For this review, take the finished solid that the model builds, in its own axes (mm). Round coordinates to 2 decimals unless told otherwise and drop trailing zeros. Write each loop counter-clockwise with the first axis right and the second up, starting at its lowest first coordinate (ties: lowest second). Pieces come first, ordered by that corner, then holes.
from build123d import *

# Parameters (mm, degrees)
F0_R     = 2.5
F1_DEPTH = 40


with BuildPart() as f1:
    # F0 (on Front) → F1 (new body)
    with BuildSketch(Plane.XZ):
        with BuildLine():
            Line((0, 37.70469), (0, 0))
            Line((0, 0), (60, 0))
            Line((60, 0), (60, 37.70469))
            ThreePointArc((60, 37.70469), (30, 45), (0, 37.70469))
        make_face()
        with Locations((7.5, 34)):
            Circle(F0_R, mode=Mode.SUBTRACT)
        with Locations((52.5, 34)):
            Circle(F0_R, mode=Mode.SUBTRACT)
    extrude(amount=F1_DEPTH)


solid = f1.part
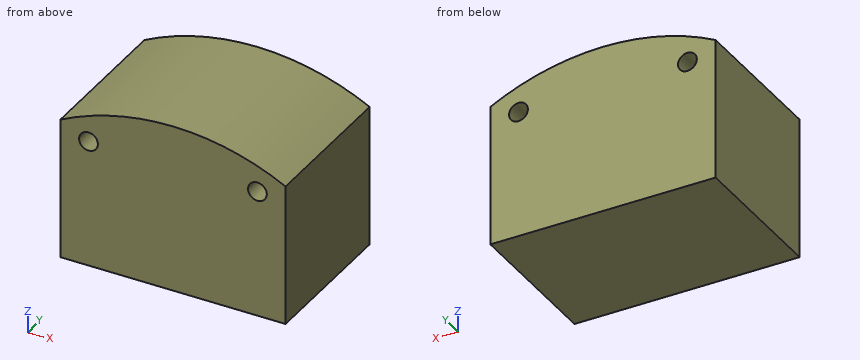
(1) We need section B-B, the plane y = -6. Give the boundary of the cut face in (x, z).
Geometry check:
outline: (0, 0) - (60, 0) - (60, 37.7) arc R65.33 ccw to (0, 37.7) - close; hole circle Ø5 at (7.5, 34); hole circle Ø5 at (52.5, 34)
(2) We need section A-A, the plane z = 34. Give the boundary of the cut face in (x, y).
Geometry check:
outline: (0, -40) - (5, -40) - (5, 0) - (0, 0) - close; (10, -40) - (50, -40) - (50, 0) - (10, 0) - close; (55, -40) - (60, -40) - (60, 0) - (55, 0) - close
(3) We need section C-C, the plane x = 52.5. Give the boundary of the cut face in (y, z).
Geometry check:
outline: (-40, 0) - (0, 0) - (0, 31.5) - (-40, 31.5) - close; (-40, 36.5) - (0, 36.5) - (0, 41) - (-40, 41) - close
(4) For line 1 along Z through (x, y) = (7.5, -20.5); line 2 along Z through (x, y) = (7, -30); line 3 along X through (y, z) = (-26.5, 39), list the stretches that pass through material, from the lowest coordinate up.
Geometry check:
line 1: z = 0 to 31.5, 36.5 to 41
line 2: z = 0 to 31.55, 36.45 to 40.82
line 3: x = 2.65 to 57.35
(5) For pin 1 Ø3 at (x, z) = (7.5, 34) entering from -Y; pin 2 Ø5 at (x, y) = (23.5, -28) entering from +Z; pin 3 Ø6 at (x, y) = (21.5, -22) entering from +Z, all flat-tipped, find the tip position at first contact; note any pin that passes through.
Geometry check:
pin 1: passes through
pin 2: stops at z = 44.88
pin 3: stops at z = 44.77
